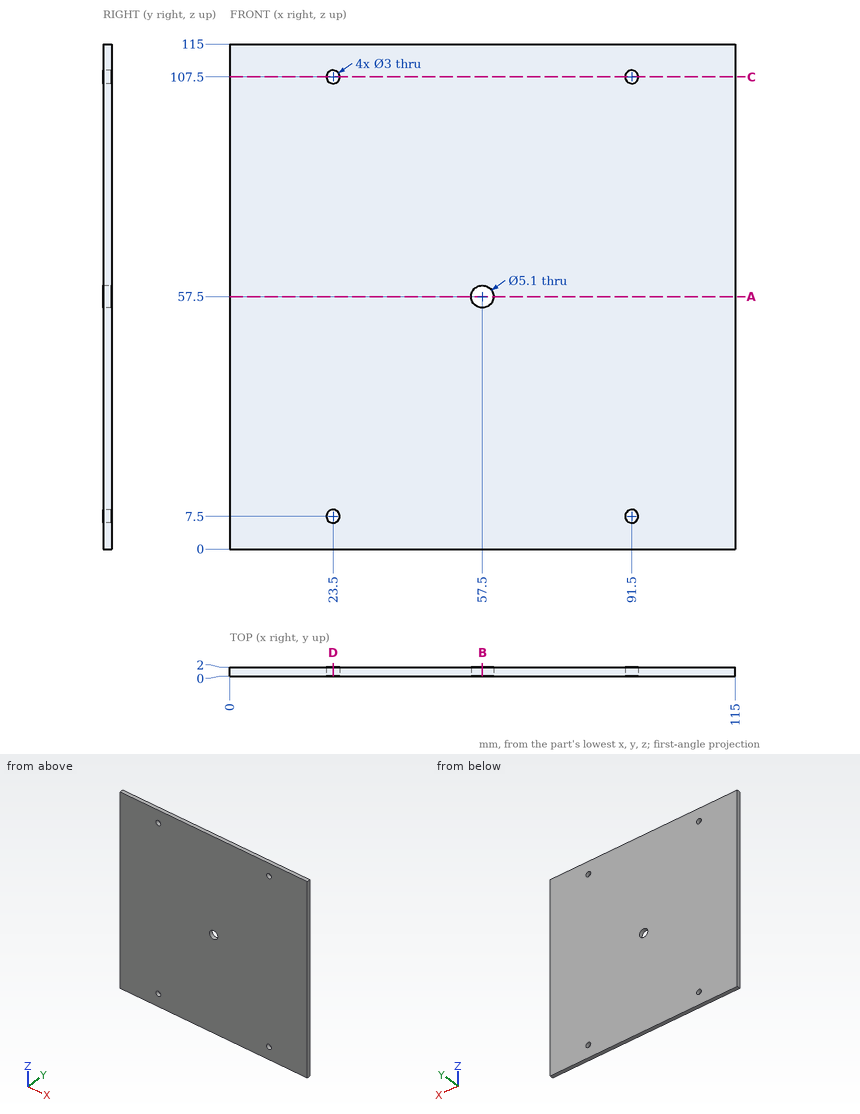
Design review of the part shown in the three views and the two pictorial views. Dimensions are in mm from the part's minimum x, y and z. Coordinates: 2 decimals unless noted, no trailing zeros. Write each loop counter-clockwise with the first axis right and the second up, starting at its lowest first coordinate (ties: lowest second). Pieces come first, ordered by that corner, then holes.
1) We need section B-B on x = 57.5. State the section outline as (y, z) points, then the cut area to 3 significant figures.
2) To check wall thickness, follow probe 1 along Z at (x, y) = (91.5, 0.95); probe 2 along X at (y, z) = (1.3, 107.5); probe 3 along X at (y, z) = (0.5, 108). State the ranges of each line that lie inside material, in increasing order.
3) Clearance check with a flat-ended pin moving along its axis: pin 1 Ø2.5 at (x, z) = (91.5, 107.5) entering from -Y. State where the tip first meets the part, or that it passes through.
4) We need section D-D on x = 23.5. State the section outline as (y, z) points.
5) We need section C-C on z = 107.5. State the section outline as (x, y) points.
6) We need section A-A on z = 57.5. State the section outline as (x, y) points, then the cut area to 3 significant figures.
Answer list:
1. outline: (0, 0) - (2, 0) - (2, 54.95) - (0, 54.95) - close; (0, 60.05) - (2, 60.05) - (2, 115) - (0, 115) - close
1. area: 220 mm2
2. probe 1: z = 0 to 6, 9 to 106, 109 to 115
2. probe 2: x = 0 to 22, 25 to 90, 93 to 115
2. probe 3: x = 0 to 22.09, 24.91 to 90.09, 92.91 to 115
3. pin 1: passes through
4. outline: (0, 0) - (2, 0) - (2, 6) - (0, 6) - close; (0, 9) - (2, 9) - (2, 106) - (0, 106) - close; (0, 109) - (2, 109) - (2, 115) - (0, 115) - close
5. outline: (0, 0) - (22, 0) - (22, 2) - (0, 2) - close; (25, 0) - (90, 0) - (90, 2) - (25, 2) - close; (93, 0) - (115, 0) - (115, 2) - (93, 2) - close
6. outline: (0, 0) - (54.95, 0) - (54.95, 2) - (0, 2) - close; (60.05, 0) - (115, 0) - (115, 2) - (60.05, 2) - close
6. area: 220 mm2
